from build123d import *

# Parameters (mm, degrees)
SKETCH1_W           = 68
SKETCH1_H           = 49.05
SKETCH1_H_2         = 15.25
SKETCH1_W_2         = 18
BOSS_EXTRUDE1_DEPTH = 60
SKETCH2_W           = 40
SKETCH2_H           = 15.25
CUT_EXTRUDE1_DEPTH  = 131.214784107
CUT_EXTRUDE2_REACH  = 132.215
CUT_EXTRUDE3_REACH  = 132.215
SKETCH5_R           = 3.25
CUT_EXTRUDE4_REACH  = 120.658
SKETCH6_R           = 2.75
SKETCH7_R           = 2.75
CUT_EXTRUDE5_DEPTH  = 131.214784107
CUT_EXTRUDE6_REACH  = 132.215
SKETCH8_R           = 3.25
CHAMFER1_SIZE       = 1
CUT_EXTRUDE8_REACH  = 132.215
SKETCH10_R          = 3.3
SKETCH10_R_2        = 2.75
SKETCH11_W          = 18.5
SKETCH11_H          = 16
BOSS_EXTRUDE2_DEPTH = 12
SKETCH12_R          = 3.25
CUT_EXTRUDE9_DEPTH  = 119.966970206
CHAMFER2_SIZE       = 1
SKETCH13_W          = 6
SKETCH13_H          = 15.25
BOSS_EXTRUDE3_DEPTH = 6
SKETCH14_W          = 6
SKETCH14_H          = 49.05
BOSS_EXTRUDE4_DEPTH = 6
SKETCH15_W          = 6
SKETCH15_H          = 49.05
SKETCH15_H_2        = 15.25
BOSS_EXTRUDE5_DEPTH = 6
BOSS_EXTRUDE6_DEPTH = 10


with BuildPart() as part:
    # Sketch1 → Boss-Extrude1 (new body)
    with BuildSketch(Plane.XY):
        Polygon((85, 0), (-29, 0), (-29, 5), (-5, 5), (-5, 52.05), (-28, 52.05), (-28, 78.3), (73, 78.3), (73, 5), (85, 5), align=None)
        with Locations((34, 27.525)):
            Rectangle(SKETCH1_W, SKETCH1_H, mode=Mode.SUBTRACT)
        with Locations((34, 64.675)):
            Rectangle(SKETCH1_W, SKETCH1_H_2, mode=Mode.SUBTRACT)
        with Locations((-14, 64.675)):
            Rectangle(SKETCH1_W_2, SKETCH1_H_2, mode=Mode.SUBTRACT)
    extrude(amount=BOSS_EXTRUDE1_DEPTH)

    # Sketch2 → Cut-Extrude1 (cut, through all)
    with BuildSketch(Plane(origin=(0, 0, 0), x_dir=(0, 0, -1), z_dir=(1, 0, 0))):
        with Locations((-30, 64.675)):
            Rectangle(SKETCH2_W, SKETCH2_H)
    extrude(amount=-CUT_EXTRUDE1_DEPTH, mode=Mode.SUBTRACT)

    # Cut-Extrude2: up to this face of the body (flat: up to its plane)
    cut_extrude2_end = Plane(part.part.faces().sort_by_distance((34, 52.05, 30))[0])
    # Sketch3 → Cut-Extrude2 (cut, up to the picked face)
    with BuildSketch(Plane(origin=(0, 78.3, 0), x_dir=(1, 0, 0), z_dir=(0, 1, 0)), mode=Mode.PRIVATE) as cut_extrude2_sk1:
        with BuildLine():
            Line((39.5, -18.5), (46.5, -18.5))
            ThreePointArc((46.5, -18.5), (58, -30), (46.5, -41.5))
            Line((46.5, -41.5), (39.5, -41.5))
            ThreePointArc((39.5, -41.5), (28, -30), (39.5, -18.5))
        make_face()
    cut_extrude2_tool1 = split(extrude(cut_extrude2_sk1.sketch, amount=-CUT_EXTRUDE2_REACH, mode=Mode.PRIVATE), bisect_by=cut_extrude2_end, keep=Keep.BOTH, mode=Mode.PRIVATE)
    # Sketch3 → Cut-Extrude2 (cut, up to the picked face)
    with BuildSketch(Plane(origin=(0, 78.3, 0), x_dir=(1, 0, 0), z_dir=(0, 1, 0)), mode=Mode.PRIVATE) as cut_extrude2_sk2:
        with BuildLine():
            Line((31, -16.25), (24, -16.25))
            ThreePointArc((24, -16.25), (22.25, -14.5), (24, -12.75))
            Line((24, -12.75), (31, -12.75))
            ThreePointArc((31, -12.75), (32.75, -14.5), (31, -16.25))
        make_face()
    cut_extrude2_tool2 = split(extrude(cut_extrude2_sk2.sketch, amount=-CUT_EXTRUDE2_REACH, mode=Mode.PRIVATE), bisect_by=cut_extrude2_end, keep=Keep.BOTH, mode=Mode.PRIVATE)
    # Sketch3 → Cut-Extrude2 (cut, up to the picked face)
    with BuildSketch(Plane(origin=(0, 78.3, 0), x_dir=(1, 0, 0), z_dir=(0, 1, 0)), mode=Mode.PRIVATE) as cut_extrude2_sk3:
        with BuildLine():
            Line((55, -16.25), (62, -16.25))
            ThreePointArc((62, -16.25), (63.75, -14.5), (62, -12.75))
            Line((62, -12.75), (55, -12.75))
            ThreePointArc((55, -12.75), (53.25, -14.5), (55, -16.25))
        make_face()
    cut_extrude2_tool3 = split(extrude(cut_extrude2_sk3.sketch, amount=-CUT_EXTRUDE2_REACH, mode=Mode.PRIVATE), bisect_by=cut_extrude2_end, keep=Keep.BOTH, mode=Mode.PRIVATE)
    # Sketch3 → Cut-Extrude2 (cut, up to the picked face)
    with BuildSketch(Plane(origin=(0, 78.3, 0), x_dir=(1, 0, 0), z_dir=(0, 1, 0)), mode=Mode.PRIVATE) as cut_extrude2_sk4:
        with BuildLine():
            Line((31, -43.75), (24, -43.75))
            ThreePointArc((24, -43.75), (22.25, -45.5), (24, -47.25))
            Line((24, -47.25), (31, -47.25))
            ThreePointArc((31, -47.25), (32.75, -45.5), (31, -43.75))
        make_face()
    cut_extrude2_tool4 = split(extrude(cut_extrude2_sk4.sketch, amount=-CUT_EXTRUDE2_REACH, mode=Mode.PRIVATE), bisect_by=cut_extrude2_end, keep=Keep.BOTH, mode=Mode.PRIVATE)
    # Sketch3 → Cut-Extrude2 (cut, up to the picked face)
    with BuildSketch(Plane(origin=(0, 78.3, 0), x_dir=(1, 0, 0), z_dir=(0, 1, 0)), mode=Mode.PRIVATE) as cut_extrude2_sk5:
        with BuildLine():
            Line((55, -43.75), (62, -43.75))
            ThreePointArc((62, -43.75), (63.75, -45.5), (62, -47.25))
            Line((62, -47.25), (55, -47.25))
            ThreePointArc((55, -47.25), (53.25, -45.5), (55, -43.75))
        make_face()
    cut_extrude2_tool5 = split(extrude(cut_extrude2_sk5.sketch, amount=-CUT_EXTRUDE2_REACH, mode=Mode.PRIVATE), bisect_by=cut_extrude2_end, keep=Keep.BOTH, mode=Mode.PRIVATE)
    add(cut_extrude2_tool1.solids().sort_by(Axis((43, 78.3, 30), (0, -1, 0)))[0], mode=Mode.SUBTRACT)
    add(cut_extrude2_tool2.solids().sort_by(Axis((27.5, 78.3, 14.5), (0, -1, 0)))[0], mode=Mode.SUBTRACT)
    add(cut_extrude2_tool3.solids().sort_by(Axis((58.5, 78.3, 14.5), (0, -1, 0)))[0], mode=Mode.SUBTRACT)
    add(cut_extrude2_tool4.solids().sort_by(Axis((27.5, 78.3, 45.5), (0, -1, 0)))[0], mode=Mode.SUBTRACT)
    add(cut_extrude2_tool5.solids().sort_by(Axis((58.5, 78.3, 45.5), (0, -1, 0)))[0], mode=Mode.SUBTRACT)

    # Sketch5 → Cut-Extrude3 (cut, up to next)
    with BuildSketch(Plane(origin=(0, 78.3, 0), x_dir=(1, 0, 0), z_dir=(0, 1, 0)), mode=Mode.PRIVATE) as cut_extrude3_sk1:
        with Locations(Location((9, -42.73, 0), (0, 0, 270))):
            Circle(SKETCH5_R)
    cut_extrude3_tool1 = extrude(cut_extrude3_sk1.sketch, amount=-CUT_EXTRUDE3_REACH, mode=Mode.PRIVATE) & part.part
    add(cut_extrude3_tool1.solids().sort_by_distance((9, 78.3, 42.73))[0], mode=Mode.SUBTRACT)

    # Sketch6 → Cut-Extrude4 (cut, up to next)
    with BuildSketch(Plane(origin=(0, 57.05, 0), x_dir=(1, 0, 0), z_dir=(0, 1, 0)), mode=Mode.PRIVATE) as cut_extrude4_sk1:
        with Locations(Location((9, -42.73, 0), (0, 0, 270))):
            Circle(SKETCH6_R)
    cut_extrude4_tool1 = extrude(cut_extrude4_sk1.sketch, amount=-CUT_EXTRUDE4_REACH, mode=Mode.PRIVATE) & part.part
    add(cut_extrude4_tool1.solids().sort_by_distance((9, 57.05, 42.73))[0], mode=Mode.SUBTRACT)

    # Sketch7 → Cut-Extrude5 (cut, through all)
    with BuildSketch(Plane(origin=(0, 78.3, 0), x_dir=(1, 0, 0), z_dir=(0, 1, 0))):
        with Locations(Location((-14, -30, 0), (0, 0, 270))):
            Circle(SKETCH7_R)
    extrude(amount=-CUT_EXTRUDE5_DEPTH, mode=Mode.SUBTRACT)

    # Sketch8 → Cut-Extrude6 (cut, up to next)
    with BuildSketch(Plane(origin=(0, 78.3, 0), x_dir=(1, 0, 0), z_dir=(0, 1, 0)), mode=Mode.PRIVATE) as cut_extrude6_sk1:
        with Locations(Location((-14, -30, 0), (0, 0, 270))):
            Circle(SKETCH8_R)
    cut_extrude6_tool1 = extrude(cut_extrude6_sk1.sketch, amount=-CUT_EXTRUDE6_REACH, mode=Mode.PRIVATE) & part.part
    add(cut_extrude6_tool1.solids().sort_by_distance((-14, 78.3, 30))[0], mode=Mode.SUBTRACT)

    # Chamfer1
    chamfer1_edges = [part.edges().sort_by_distance(p)[0] for p in [
        (9, 78.3, 39.48),
        (-14, 78.3, 26.75),
    ]]
    chamfer(chamfer1_edges, length=CHAMFER1_SIZE)

    # Sketch10 → Cut-Extrude8 (cut, up to next)
    with BuildSketch(Plane.XZ, mode=Mode.PRIVATE) as cut_extrude8_sk1:
        with Locations((-21, 45)):
            Circle(SKETCH10_R)
    cut_extrude8_tool1 = extrude(cut_extrude8_sk1.sketch, amount=-CUT_EXTRUDE8_REACH, mode=Mode.PRIVATE) & part.part
    # Sketch10 → Cut-Extrude8 (cut, up to next)
    with BuildSketch(Plane.XZ, mode=Mode.PRIVATE) as cut_extrude8_sk2:
        with Locations((-21, 15)):
            Circle(SKETCH10_R)
    cut_extrude8_tool2 = extrude(cut_extrude8_sk2.sketch, amount=-CUT_EXTRUDE8_REACH, mode=Mode.PRIVATE) & part.part
    # Sketch10 → Cut-Extrude8 (cut, up to next)
    with BuildSketch(Plane.XZ, mode=Mode.PRIVATE) as cut_extrude8_sk3:
        with Locations((79, 15)):
            Circle(SKETCH10_R_2)
    cut_extrude8_tool3 = extrude(cut_extrude8_sk3.sketch, amount=-CUT_EXTRUDE8_REACH, mode=Mode.PRIVATE) & part.part
    # Sketch10 → Cut-Extrude8 (cut, up to next)
    with BuildSketch(Plane.XZ, mode=Mode.PRIVATE) as cut_extrude8_sk4:
        with Locations((79, 45)):
            Circle(SKETCH10_R_2)
    cut_extrude8_tool4 = extrude(cut_extrude8_sk4.sketch, amount=-CUT_EXTRUDE8_REACH, mode=Mode.PRIVATE) & part.part
    add(cut_extrude8_tool1.solids().sort_by_distance((-21, 0, 45))[0], mode=Mode.SUBTRACT)
    add(cut_extrude8_tool2.solids().sort_by_distance((-21, 0, 15))[0], mode=Mode.SUBTRACT)
    add(cut_extrude8_tool3.solids().sort_by_distance((79, 0, 15))[0], mode=Mode.SUBTRACT)
    add(cut_extrude8_tool4.solids().sort_by_distance((79, 0, 45))[0], mode=Mode.SUBTRACT)

    # Sketch11 → Boss-Extrude2 (add)
    with BuildSketch(Plane.XZ.offset(-52.05)):
        with Locations((9.25, 30)):
            Rectangle(SKETCH11_W, SKETCH11_H)
    extrude(amount=BOSS_EXTRUDE2_DEPTH)

    # Sketch12 → Cut-Extrude9 (cut, through all)
    with BuildSketch(Plane(origin=(18.5, 0, 0), x_dir=(0, 0, -1), z_dir=(1, 0, 0))):
        with Locations((-29.33403853, 46.549471103)):
            Circle(SKETCH12_R)
    extrude(amount=-CUT_EXTRUDE9_DEPTH, mode=Mode.SUBTRACT)

    # Chamfer2
    chamfer2_edges = [part.edges().sort_by_distance(p)[0] for p in [
        (-5, 46.549471103, 32.58403853),
    ]]
    chamfer(chamfer2_edges, length=CHAMFER2_SIZE)

    # Sketch13 → Boss-Extrude3 (add)
    with BuildSketch(Plane.XY.offset(60)):
        with Locations((34, 64.675)):
            Rectangle(SKETCH13_W, SKETCH13_H)
    extrude(amount=-BOSS_EXTRUDE3_DEPTH)

    # Sketch14 → Boss-Extrude4 (add)
    with BuildSketch(Plane.XY.offset(60)):
        with Locations((23, 27.525)):
            Rectangle(SKETCH14_W, SKETCH14_H)
        with Locations((45, 27.525)):
            Rectangle(SKETCH14_W, SKETCH14_H)
    extrude(amount=-BOSS_EXTRUDE4_DEPTH)

    # Sketch15 → Boss-Extrude5 (add)
    with BuildSketch(Plane(origin=(0, 0, 0), x_dir=(-1, 0, 0), z_dir=(0, 0, -1))):
        with Locations((-23, 27.525)):
            Rectangle(SKETCH15_W, SKETCH15_H)
        with Locations((-34, 64.675)):
            Rectangle(SKETCH15_W, SKETCH15_H_2)
    extrude(amount=-BOSS_EXTRUDE5_DEPTH)

    # Sketch16 → Boss-Extrude6 (add)
    with BuildSketch(Plane(origin=(0, 0, 0), x_dir=(-1, 0, 0), z_dir=(0, 0, -1))):
        Polygon((28, 52.05), (5, 29.05), (5, 52.05), align=None)
    extrude(amount=-BOSS_EXTRUDE6_DEPTH)


solid = part.part
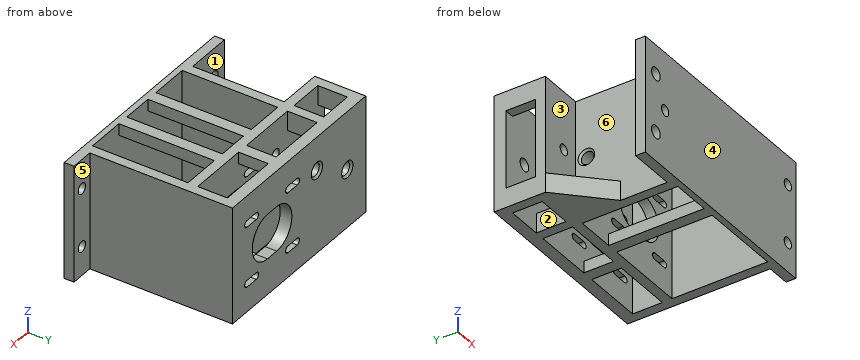
The model under review builds one solid part; all positions refer to its coordinate system, in mm. Face numbers are marked on the shaded views. A direction names the side the tool comes from. Round coordinates to 2 decimals unless told otherwise and drop trailing zeros. Loops run counter-clockwise (first coordinate to the right, second up) from the corner with the lowest first, then second, coordinate; pieces in that order, holes last. Notation, with made-up numbers: (48.25, 4.25) -> (66.25, 4.25) arc R9 cw to (66.25, 17.25) -> close; hole circle Ø1 at (-6, -6.5). An arc over 180 degrees is marked (long way). Return JSON: item names as keys, results as strings.
(1) For line 1 (Y direction, x = 29, z = 57); line 2 (Z direction, x = -21, y = 2.4); line 3 (Y direction, x = -24, z = 31.5), list the stretches that pass through material, from the lowest coordinate up.
Solved:
{"line 1": "0 to 3, 52.05 to 57.05, 72.3 to 78.3", "line 2": "0 to 11.7, 18.3 to 41.7, 48.3 to 60", "line 3": "0 to 5, 52.05 to 57.05, 72.3 to 78.3"}
(2) The part is to be moulded in two halves that separate along Y. For the marked faces 4, 5 and 6, say which applies: released by +Y, released by -Y, zero draft, split by the parting line, or undercut.
Solved:
{"face 4": "released by -Y", "face 5": "released by +Y", "face 6": "undercut"}
(3) Add section D-D on x = 17. Write out the cut boundary in (y, z), plus the area to 3 significant figures.
Solved:
{"outline": "(0, 0) -> (3, 0) -> (3, 60) -> (0, 60) -> close; (40.05, 22) -> (52.05, 22) -> (52.05, 0) -> (57.05, 0) -> (57.05, 60) -> (52.05, 60) -> (52.05, 38) -> (40.05, 38) -> close; (72.3, 0) -> (78.3, 0) -> (78.3, 60) -> (72.3, 60) -> close; hole circle Ø6.5 at (46.55, 29.33)", "area": "999 mm2"}
(4) Add section B-B on x = -21. Write out the cut boundary in (y, z).
Solved:
{"outline": "(0, 0) -> (5, 0) -> (5, 11.7) -> (0, 11.7) -> close; (0, 18.3) -> (5, 18.3) -> (5, 41.7) -> (0, 41.7) -> close; (0, 48.3) -> (5, 48.3) -> (5, 60) -> (0, 60) -> close; (45.05, 0) -> (57.05, 0) -> (57.05, 60) -> (52.05, 60) -> (52.05, 10) -> (45.05, 10) -> close; (72.3, 0) -> (78.3, 0) -> (78.3, 60) -> (72.3, 60) -> close"}
(5) For pin 1 (5 mm diameter, centred on x = 28, z = 32, fed in from -Y); pin 2 (1.8 mm diameter, centred on x = 44, y = 16.5, fed in from -Z); pin 3 (5 mm diameter, centred on y = 28, z = 2, fed in from +X); pin 4 (7 mm diameter, centred on x = -14, z = 30, fed in from +Y), all flat-tipped, find the tip position at first contact; note any pin that passes through.
Solved:
{"pin 1": "y = 0", "pin 2": "z = 54", "pin 3": "x = 73", "pin 4": "y = 77.55"}
(6) Add section C-C on y = 22. Write out the cut boundary in (x, z), plus the area to 3 significant figures.
Solved:
{"outline": "(-5, 0) -> (0, 0) -> (0, 60) -> (-5, 60) -> close; (20, 0) -> (26, 0) -> (26, 6) -> (20, 6) -> close; (20, 54) -> (26, 54) -> (26, 60) -> (20, 60) -> close; (42, 54) -> (48, 54) -> (48, 60) -> (42, 60) -> close; (68, 0) -> (73, 0) -> (73, 60) -> (68, 60) -> close", "area": "708 mm2"}
(7) Add section A-A on x = 79. Write out the cut boundary in (y, z).
Solved:
{"outline": "(0, 0) -> (5, 0) -> (5, 12.25) -> (0, 12.25) -> close; (0, 17.75) -> (5, 17.75) -> (5, 42.25) -> (0, 42.25) -> close; (0, 47.75) -> (5, 47.75) -> (5, 60) -> (0, 60) -> close"}
(8) For the marked faces 1, 2 and 3, list the 3-axis set-ups (+Z, -Z, +X, -X, +Y, -Y) from which the entire face can be reached by the end or side of a thin tool; tool diameter is ignored.
Solved:
{"face 1": "+Z, -Z, -X", "face 2": "+Z, -Z", "face 3": "+Z, -X"}
